from build123d import *

# Parameters (mm, degrees)
F0_W     = 32
F0_H     = 50
F1_DEPTH = 15
F2_SIZE  = 4.5
F3_W     = 44.522483
F3_H     = 61.777794
F4_DEPTH = 8.5
F6_DEPTH = 3
F8_DEPTH = 5


with BuildPart() as f1:
    # F0 (on Front) → F1 (new body)
    with BuildSketch(Plane.XZ):
        with Locations((16, 25)):
            Rectangle(F0_W, F0_H)
    extrude(amount=F1_DEPTH)

    # F2
    f2_edges = [f1.edges().sort_by_distance(p)[0] for p in [
        (0, -7.5, 50),
        (0, -7.5, 0),
        (0, 0, 25),
        (0, -15, 25),
        (16, 0, 0),
        (32, 0, 25),
        (16, 0, 50),
        (32, -7.5, 50),
        (16, -15, 50),
        (32, -7.5, 0),
        (32, -15, 25),
        (16, -15, 0),
    ]]
    chamfer(f2_edges, length=F2_SIZE)

    # F3 (on face) → F4 (cut)
    with BuildSketch(Plane.XZ.offset(15)):
        with Locations((18.562658, 27.901019)):
            Rectangle(F3_W, F3_H)
    extrude(amount=-F4_DEPTH, mode=Mode.SUBTRACT)

    # F5 (on face) → F6 (join)
    with BuildSketch(Plane.XZ.offset(6.5)):
        Polygon((2.2, 4.5), (4.5, 2.2), (27.5, 2.2), (29.8, 4.5), (29.8, 45.5), (27.5, 47.8), (4.5, 47.8), (2.2, 45.5), align=None)
    extrude(amount=F6_DEPTH)

    # F7 (on face) → F8 (cut)
    with BuildSketch(Plane.XZ.offset(9.5)):
        Polygon((4.2, 4.5), (4.5, 4.2), (27.5, 4.2), (27.8, 4.5), (27.8, 45.5), (27.5, 45.8), (4.5, 45.8), (4.2, 45.5), align=None)
    extrude(amount=-F8_DEPTH, mode=Mode.SUBTRACT)


solid = f1.part
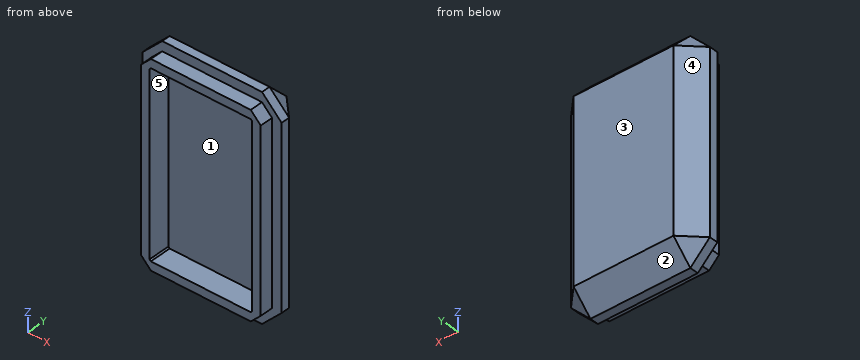
Build history of the part. All positions in model axes, mm. Face numbers are marked on the shaded views. A direction names the side the tool comes from. Give positions to 0.01 mm unless a question says otherwise; leave off trailing zeros. Loops run counter-clockwise (first coordinate to the right, second up) from the corner with the lowest first, then second, coordinate; pieces in that order, holes last. Notation, with made-up numbers: (64.25, 4.5) -> (109.25, 4.5) arc R18 ccw to (109.25, 32.5) -> close; hole circle Ø5 at (57, 87). An arc over 180 degrees is marked (long way). Answer in a Markdown table with one row per item.
Item 1: Slice it at A-A on y = -7. Write the cut outline in (x, z).
Findings below:
| item | result |
|---|---|
| outline | (2.2, 4.5) -> (4.5, 2.2) -> (27.5, 2.2) -> (29.8, 4.5) -> (29.8, 45.5) -> (27.5, 47.8) -> (4.5, 47.8) -> (2.2, 45.5) -> close; hole (4.2, 4.5) -> (4.5, 4.2) -> (27.5, 4.2) -> (27.8, 4.5) -> (27.8, 45.5) -> (27.5, 45.8) -> (4.5, 45.8) -> (4.2, 45.5) -> close |
Item 2: Probe line 1 along X through (y, z) = (-5.5, 16); line 2 along Z through (x, y) = (25.5, -5.25); line 3 along Z through (x, y) = (19.5, -8). List the from-to ranges inside material, lowest first. Write a range as [from, to].
Findings below:
| item | result |
|---|---|
| line 1 | x = [0, 4.2], [27.8, 32] |
| line 2 | z = [0, 4.2], [45.8, 50] |
| line 3 | z = [2.2, 4.2], [45.8, 47.8] |
Item 3: Slice it at C-C on z = 35. Write the cut outline in (x, y).
Findings below:
| item | result |
|---|---|
| outline | (0, -6.5) -> (2.2, -6.5) -> (2.2, -9.5) -> (4.2, -9.5) -> (4.2, -4.5) -> (27.8, -4.5) -> (27.8, -9.5) -> (29.8, -9.5) -> (29.8, -6.5) -> (32, -6.5) -> (32, -4.5) -> (27.5, 0) -> (4.5, 0) -> (0, -4.5) -> close |
Item 4: Slice it at B-B on x = 5.5. Write the cut outline in (y, z).
Findings below:
| item | result |
|---|---|
| outline | (-9.5, 2.2) -> (-6.5, 2.2) -> (-6.5, 0) -> (-4.5, 0) -> (0, 4.5) -> (0, 45.5) -> (-4.5, 50) -> (-6.5, 50) -> (-6.5, 47.8) -> (-9.5, 47.8) -> (-9.5, 45.8) -> (-4.5, 45.8) -> (-4.5, 4.2) -> (-9.5, 4.2) -> close |
Item 5: Mould opens along X. For the marked faces 3, 4 and 5 say: pulls with the +X half, pulls with the -X half, needs draft (parallel to the pull), parting line crosses it, or undercut.
Findings below:
| item | result |
|---|---|
| face 3 | needs draft |
| face 4 | pulls with the -X half |
| face 5 | undercut |
Item 6: Flat gauge pins, fed straight in: P1, Ø5, axis at x = 21, z = 16.5, coming from the -Y side; P2, Ø1.5, axis at y = -7.5, z = 36, coming from the +X side; P3, Ø1.5, axis at y = -7.5, z = 15.5, coming from the -X side. Where does each tip first touch, or does it go through?
Findings below:
| item | result |
|---|---|
| P1 | stops at y = -4.5 |
| P2 | stops at x = 29.8 |
| P3 | stops at x = 2.2 |
Item 7: Slice it at D-D on y = -2.5. Write the cut outline in (x, z).
Findings below:
| item | result |
|---|---|
| outline | (2, 4.5) -> (4.5, 2) -> (27.5, 2) -> (30, 4.5) -> (30, 45.5) -> (27.5, 48) -> (4.5, 48) -> (2, 45.5) -> close |
Item 8: Tool access for the marked faces 1 and 2: list every direction of +Z, -Z, +X, -X, +Y, -Y with a clear straight run to the whole face (end or side of a thin tool).
Findings below:
| item | result |
|---|---|
| face 1 | -Y |
| face 2 | -Z, +X, -X, +Y |
